Here's how the part is built. I have some questions about the finished solid (model axes, mm). Coordinates: 2 decimals unless noted, no trailing zeros. Write each loop counter-clockwise with the first axis right and the second up, starting at its lowest first coordinate (ties: lowest second). Pieces come first, ordered by that corner, then holes. Notation, with made-up numbers: M -2.5,20 L 5.5,20 A32 ccw 5.5,54 Z; hole C -19,-6.75 d10. An arc over 180 degrees is marked long. Use one line per item in the form item = value. Start each with the question number.
1. I'm going to push a flat-ended pin straight in: pin 1 Ø21 at (x, z) = (18.1, -231.32) entering from -Y. Where does the tip first touch, or does it pass through?
2. Please list where these lines run through material, in increasing order: line 1 along X through (y, z) = (1, 99.5); line 2 along X through (y, z) = (-4.5, 177.5); line 3 along X through (y, z) = (-2.75, 65). Write a range as [from, to].
3. I want a section at A-A, the plane z = 0. List the corners of the cut face in (x, y) for me, plus the area to 3 significant figures.
4. I want a section at B-B, the plane y = -2.75. Count the separate pieces of the cut face and the enclosed holes in it, plus the area to 3 significant figures.
5. I want a section at C-C, the plane z = -74. List the corners of the cut face in (x, y) for me.
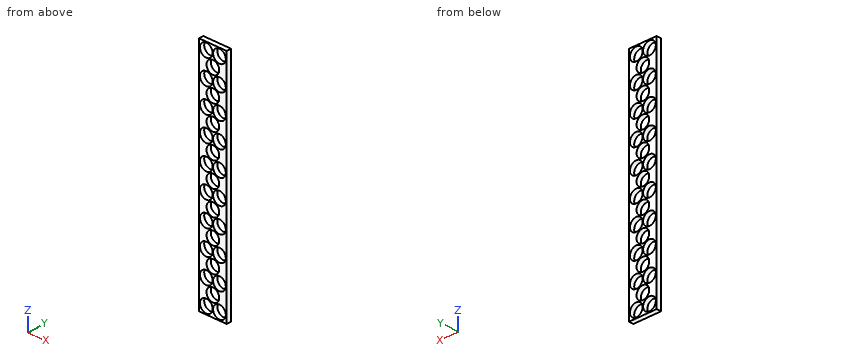
from build123d import *

# Parameters (mm, degrees)
SKETCH1_W           = 76.2
SKETCH1_H           = 12.7
BOSS_EXTRUDE1_DEPTH = 317.5
CUT_EXTRUDE1_REACH  = 322.03
SKETCH2_R           = 17.4625
LPATTERN1_COUNT     = 5
LPATTERN1_PITCH     = 66.173358604
MIRROR1_START       = -6.35
MIRROR1_OUTLINE_R   = 17.4625
MIRROR1_DEPTH       = 12.7


# Read off the part's stored shape, not the designer's step: Mirror1
with BuildPart() as part:
    # Sketch1 → Boss-Extrude1 (new, symmetric)
    with BuildSketch(Plane.XY):
        Rectangle(SKETCH1_W, SKETCH1_H)
    extrude(amount=BOSS_EXTRUDE1_DEPTH, both=True)

    # Sketch2 → Cut-Extrude1 (cut, up to next)
    with BuildSketch(Plane(origin=(0, 6.35, 0), x_dir=(1, 0, 0), z_dir=(0, 1, 0)), mode=Mode.PRIVATE) as cut_extrude1_sk1:
        with Locations(Location((-18.0975, -297.4975, 0), (0, 0, 180))):
            Circle(SKETCH2_R)
    cut_extrude1_tool1 = extrude(cut_extrude1_sk1.sketch, amount=-CUT_EXTRUDE1_REACH, mode=Mode.PRIVATE) & part.part
    # Sketch2 → Cut-Extrude1 (cut, up to next)
    with BuildSketch(Plane(origin=(0, 6.35, 0), x_dir=(1, 0, 0), z_dir=(0, 1, 0)), mode=Mode.PRIVATE) as cut_extrude1_sk2:
        with Locations(Location((0, -264.693434417, 0), (0, 0, 180))):
            Circle(SKETCH2_R)
    cut_extrude1_tool2 = extrude(cut_extrude1_sk2.sketch, amount=-CUT_EXTRUDE1_REACH, mode=Mode.PRIVATE) & part.part
    # Sketch2 → Cut-Extrude1 (cut, up to next)
    with BuildSketch(Plane(origin=(0, 6.35, 0), x_dir=(1, 0, 0), z_dir=(0, 1, 0)), mode=Mode.PRIVATE) as cut_extrude1_sk3:
        with Locations(Location((18.0975, -297.4975, 0), (0, 0, 180))):
            Circle(SKETCH2_R)
    cut_extrude1_tool3 = extrude(cut_extrude1_sk3.sketch, amount=-CUT_EXTRUDE1_REACH, mode=Mode.PRIVATE) & part.part
    cut_extrude1_1 = cut_extrude1_tool1.solids().sort_by_distance((-18.0975, 6.35, 297.4975))[0]
    add(cut_extrude1_1, mode=Mode.SUBTRACT)
    cut_extrude1_2 = cut_extrude1_tool2.solids().sort_by_distance((0, 6.35, 264.693434))[0]
    add(cut_extrude1_2, mode=Mode.SUBTRACT)
    cut_extrude1_3 = cut_extrude1_tool3.solids().sort_by_distance((18.0975, 6.35, 297.4975))[0]
    add(cut_extrude1_3, mode=Mode.SUBTRACT)
    cut_extrude1 = cut_extrude1_1 + cut_extrude1_2 + cut_extrude1_3  # Cut-Extrude1 as one shape, for the pattern or mirror that repeats it

    # LPattern1: Cut-Extrude1 ×5
    with Locations(*[(0, 0, -i * LPATTERN1_PITCH) for i in range(1, LPATTERN1_COUNT)]):
        add(cut_extrude1, mode=Mode.SUBTRACT)

    # Mirror1 outline → Mirror1 (cut)
    with BuildSketch(Plane(origin=(0, 0, 0), x_dir=(1, 0, 0), z_dir=(0, 1, 0)).offset(MIRROR1_START)):
        with Locations((-18.0975, 297.4975)):
            Circle(MIRROR1_OUTLINE_R)
        with Locations((-18.0975, 32.804065583)):
            Circle(MIRROR1_OUTLINE_R)
        with Locations((18.0975, 98.977424187)):
            Circle(MIRROR1_OUTLINE_R)
        with Locations((-18.0975, 98.977424187)):
            Circle(MIRROR1_OUTLINE_R)
        with Locations((0, 66.173358604)):
            Circle(MIRROR1_OUTLINE_R)
        with Locations((18.0975, 32.804065583)):
            Circle(MIRROR1_OUTLINE_R)
        with Locations((-18.0975, 231.324141396)):
            Circle(MIRROR1_OUTLINE_R)
        with Locations((0, 198.520075813)):
            Circle(MIRROR1_OUTLINE_R)
        with Locations((0, 264.693434417)):
            Circle(MIRROR1_OUTLINE_R)
        with Locations((18.0975, 297.4975)):
            Circle(MIRROR1_OUTLINE_R)
        with Locations((0, 132.346717209)):
            Circle(MIRROR1_OUTLINE_R)
        with Locations((18.0975, 165.150782791)):
            Circle(MIRROR1_OUTLINE_R)
        with Locations((-18.0975, 165.150782791)):
            Circle(MIRROR1_OUTLINE_R)
        with Locations((18.0975, 231.324141396)):
            Circle(MIRROR1_OUTLINE_R)
    extrude(amount=MIRROR1_DEPTH, mode=Mode.SUBTRACT)


solid = part.part
Answer list:
q1.pin_1 = through
q2.line_1 = [-38.1, -35.55], [-0.64, 0.64], [35.55, 38.1]
q2.line_2 = [-38.1, -30.44], [-5.75, 5.75], [30.44, 38.1]
q2.line_3 = [-38.1, -17.42], [17.42, 38.1]
q3.outline = M -38.1,-6.35 L -17.46,-6.35 L -17.46,6.35 L -38.1,6.35 Z; M 17.46,-6.35 L 38.1,-6.35 L 38.1,6.35 L 17.46,6.35 Z
q3.area = 524 mm²
q4.separate_pieces = 1
q4.enclosed_holes = 29
q4.area = 20,600 mm²
q5.outline = M -38.1,-6.35 L -15.61,-6.35 L -15.61,6.35 L -38.1,6.35 Z; M 15.61,-6.35 L 38.1,-6.35 L 38.1,6.35 L 15.61,6.35 Z
